```python
from build123d import *

# Parameters (mm, degrees)
BOSS_EXTRUDE3_DEPTH      = 4
BOSS_EXTRUDE3_DEPTH_BACK = 13
SKETCH1_R                = 2.5
SKETCH1_R_2              = 4.5
SKETCH1_R_3              = 2
SKETCH1_R_4              = 1
BOSS_EXTRUDE4_DEPTH      = 0.0001
BOSS_EXTRUDE4_DEPTH_BACK = 1
SKETCH1_3_R              = 1
SKETCH1_8_R              = 1
BOSS_EXTRUDE6_DEPTH      = 7
SKETCH1_9_R              = 2
BOSS_EXTRUDE7_DEPTH      = 11
SKETCH1_11_R             = 4.5
BOSS_EXTRUDE10_DEPTH     = 8
SKETCH1_12_R             = 4.5
SKETCH1_12_R_2           = 2.5
SKETCH1_12_R_3           = 1
BOSS_EXTRUDE11_DEPTH     = 6


with BuildPart() as part:
    # Sketch1 → Boss-Extrude3 (new, two sides: drawn at the far end of the back side and taken through both)
    # profile 1 of 14: a face of its own
    with BuildSketch(Plane(origin=(0, 0, 0), x_dir=(1, 0, 0), z_dir=(0, 1, 0)).offset(-BOSS_EXTRUDE3_DEPTH_BACK)):
        with BuildLine():
            ThreePointArc((-1.694444444, -2.401613398), (-3.327128661, -3.940638292), (-5.5, -4.5))
            Line((-5.5, -4.5), (10, -4.5))
            Line((10, -4.5), (10, 4.5))
            Line((10, 4.5), (-5.5, 4.5))
            ThreePointArc((-5.5, 4.5), (-3.327128661, 3.940638292), (-1.694444444, 2.401613398))
            ThreePointArc((-1.694444444, 2.401613398), (0.502313031, 1.998263135), (1.5, 0))
            ThreePointArc((1.5, 0), (0.502313031, -1.998263135), (-1.694444444, -2.401613398))
        make_face()
    # profile 2 of 14: a face of its own
    with BuildSketch(Plane(origin=(0, 0, 0), x_dir=(1, 0, 0), z_dir=(0, 1, 0)).offset(-BOSS_EXTRUDE3_DEPTH_BACK)):
        with BuildLine():
            Line((-10, 0), (-10, -4.5))
            Line((-10, -4.5), (-5.5, -4.5))
            ThreePointArc((-5.5, -4.5), (-8.681980515, -3.181980515), (-10, 0))
        make_face()
    # profile 3 of 14: a face of its own
    with BuildSketch(Plane(origin=(0, 0, 0), x_dir=(1, 0, 0), z_dir=(0, 1, 0)).offset(-BOSS_EXTRUDE3_DEPTH_BACK)):
        with BuildLine():
            Line((-10, 4.5), (-10, 0))
            ThreePointArc((-10, 0), (-8.681980515, 3.181980515), (-5.5, 4.5))
            Line((-5.5, 4.5), (-10, 4.5))
        make_face()
    # profile 4 of 14: a face of its own
    with BuildSketch(Plane(origin=(0, 0, 0), x_dir=(1, 0, 0), z_dir=(0, 1, 0)).offset(-BOSS_EXTRUDE3_DEPTH_BACK)):
        with Locations((-1, 0)):
            Circle(SKETCH1_R)
    # profile 5 of 14: a face of its own
    with BuildSketch(Plane(origin=(0, 0, 0), x_dir=(1, 0, 0), z_dir=(0, 1, 0)).offset(-BOSS_EXTRUDE3_DEPTH_BACK)):
        with Locations((-5.5, 0)):
            Circle(SKETCH1_R_2)
        with Locations((-5.5, 0)):
            Circle(SKETCH1_R_3, mode=Mode.SUBTRACT)
    # profile 6 of 14: a face of its own
    with BuildSketch(Plane(origin=(0, 0, 0), x_dir=(1, 0, 0), z_dir=(0, 1, 0)).offset(-BOSS_EXTRUDE3_DEPTH_BACK)):
        with Locations((-5.5, 0)):
            Circle(SKETCH1_R_3)
    # profile 7 of 14: a face of its own
    with BuildSketch(Plane(origin=(0, 0, 0), x_dir=(1, 0, 0), z_dir=(0, 1, 0)).offset(-BOSS_EXTRUDE3_DEPTH_BACK)):
        with Locations((-5.5, 0)):
            Circle(SKETCH1_R_2)
    # profile 8 of 14: a face of its own
    with BuildSketch(Plane(origin=(0, 0, 0), x_dir=(1, 0, 0), z_dir=(0, 1, 0)).offset(-BOSS_EXTRUDE3_DEPTH_BACK)):
        with Locations((-1, 0)):
            Circle(SKETCH1_R)
        with Locations((-1, 0)):
            Circle(SKETCH1_R_4, mode=Mode.SUBTRACT)
    # profile 9 of 14: a face of its own
    with BuildSketch(Plane(origin=(0, 0, 0), x_dir=(1, 0, 0), z_dir=(0, 1, 0)).offset(-BOSS_EXTRUDE3_DEPTH_BACK)):
        with Locations((-5.5, 0)):
            Circle(SKETCH1_R_2)
    # profile 10 of 14: a face of its own
    with BuildSketch(Plane(origin=(0, 0, 0), x_dir=(1, 0, 0), z_dir=(0, 1, 0)).offset(-BOSS_EXTRUDE3_DEPTH_BACK)):
        with Locations((-1, 0)):
            Circle(SKETCH1_R)
        with Locations((-1, 0)):
            Circle(SKETCH1_R_4, mode=Mode.SUBTRACT)
    # profile 11 of 14: a face of its own
    with BuildSketch(Plane(origin=(0, 0, 0), x_dir=(1, 0, 0), z_dir=(0, 1, 0)).offset(-BOSS_EXTRUDE3_DEPTH_BACK)):
        with Locations((-5.5, 0)):
            Circle(SKETCH1_R_2)
    # profile 12 of 14: a face of its own
    with BuildSketch(Plane(origin=(0, 0, 0), x_dir=(1, 0, 0), z_dir=(0, 1, 0)).offset(-BOSS_EXTRUDE3_DEPTH_BACK)):
        with Locations((-1, 0)):
            Circle(SKETCH1_R_4)
    # profile 13 of 14: a face of its own
    with BuildSketch(Plane(origin=(0, 0, 0), x_dir=(1, 0, 0), z_dir=(0, 1, 0)).offset(-BOSS_EXTRUDE3_DEPTH_BACK)):
        with Locations((-5.5, 0)):
            Circle(SKETCH1_R_2)
    # profile 14 of 14: a face of its own
    with BuildSketch(Plane(origin=(0, 0, 0), x_dir=(1, 0, 0), z_dir=(0, 1, 0)).offset(-BOSS_EXTRUDE3_DEPTH_BACK)):
        with Locations((-1, 0)):
            Circle(SKETCH1_R_4)
    extrude(amount=BOSS_EXTRUDE3_DEPTH + BOSS_EXTRUDE3_DEPTH_BACK)

    # Sketch1_3 → Boss-Extrude4 (add, two sides: drawn at the far end of the back side and taken through both)
    # profile 1 of 2: a face of its own
    with BuildSketch(Plane(origin=(0, 0, 0), x_dir=(1, 0, 0), z_dir=(0, 1, 0)).offset(-BOSS_EXTRUDE4_DEPTH_BACK)):
        with BuildLine():
            Line((-14, -4.5), (-10, -4.5))
            Line((-10, -4.5), (-10, 4.5))
            Line((-10, 4.5), (-14, 4.5))
            ThreePointArc((-14, 4.5), (-16.985823737, 0), (-14, -4.5))
        make_face()
        with Locations(Location((-13, 0, 0), (0, 0, 270))):
            Circle(SKETCH1_3_R, mode=Mode.SUBTRACT)
    # profile 2 of 2: a face of its own
    with BuildSketch(Plane(origin=(0, 0, 0), x_dir=(1, 0, 0), z_dir=(0, 1, 0)).offset(-BOSS_EXTRUDE4_DEPTH_BACK)):
        with BuildLine():
            Line((10, 4.5), (10, -4.5))
            Line((10, -4.5), (14, -4.5))
            ThreePointArc((14, -4.5), (17.054182563, 0), (14, 4.5))
            Line((14, 4.5), (10, 4.5))
        make_face()
        with Locations(Location((13, 0, 0), (0, 0, 270))):
            Circle(SKETCH1_3_R, mode=Mode.SUBTRACT)
    extrude(amount=BOSS_EXTRUDE4_DEPTH + BOSS_EXTRUDE4_DEPTH_BACK)

    # Sketch1_8 → Boss-Extrude6 (add)
    with BuildSketch(Plane(origin=(0, 0, 0), x_dir=(1, 0, 0), z_dir=(0, 1, 0))):
        with Locations(Location((-1, 0, 0), (0, 0, 270))):
            Circle(SKETCH1_8_R)
    extrude(amount=BOSS_EXTRUDE6_DEPTH)

    # Sketch1_9 → Boss-Extrude7 (add)
    with BuildSketch(Plane(origin=(0, 0, 0), x_dir=(1, 0, 0), z_dir=(0, 1, 0))):
        with Locations(Location((-5.5, 0, 0), (0, 0, 270))):
            Circle(SKETCH1_9_R)
    extrude(amount=BOSS_EXTRUDE7_DEPTH)

    # Sketch1_11 → Boss-Extrude10 (add)
    with BuildSketch(Plane(origin=(0, 0, 0), x_dir=(1, 0, 0), z_dir=(0, 1, 0))):
        with Locations(Location((-5.5, 0, 0), (0, 0, 270))):
            Circle(SKETCH1_11_R)
    extrude(amount=BOSS_EXTRUDE10_DEPTH)

    # Sketch1_12 → Boss-Extrude11 (add)
    # profile 1 of 8: a face of its own
    with BuildSketch(Plane(origin=(0, 0, 0), x_dir=(1, 0, 0), z_dir=(0, 1, 0))):
        with Locations(Location((-5.5, 0, 0), (0, 0, 270))):
            Circle(SKETCH1_12_R)
    # profile 2 of 8: a face of its own
    with BuildSketch(Plane(origin=(0, 0, 0), x_dir=(1, 0, 0), z_dir=(0, 1, 0))):
        with Locations((-1, 0)):
            Circle(SKETCH1_12_R_2)
        with Locations((-1, 0)):
            Circle(SKETCH1_12_R_3, mode=Mode.SUBTRACT)
    # profile 3 of 8: a face of its own
    with BuildSketch(Plane(origin=(0, 0, 0), x_dir=(1, 0, 0), z_dir=(0, 1, 0))):
        with Locations(Location((-5.5, 0, 0), (0, 0, 270))):
            Circle(SKETCH1_12_R)
    # profile 4 of 8: a face of its own
    with BuildSketch(Plane(origin=(0, 0, 0), x_dir=(1, 0, 0), z_dir=(0, 1, 0))):
        with Locations(Location((-5.5, 0, 0), (0, 0, 270))):
            Circle(SKETCH1_12_R)
    # profile 5 of 8: a face of its own
    with BuildSketch(Plane(origin=(0, 0, 0), x_dir=(1, 0, 0), z_dir=(0, 1, 0))):
        with Locations((-1, 0)):
            Circle(SKETCH1_12_R_2)
        with Locations((-1, 0)):
            Circle(SKETCH1_12_R_3, mode=Mode.SUBTRACT)
    # profile 6 of 8: a face of its own
    with BuildSketch(Plane(origin=(0, 0, 0), x_dir=(1, 0, 0), z_dir=(0, 1, 0))):
        with Locations((-1, 0)):
            Circle(SKETCH1_12_R_3)
    # profile 7 of 8: a face of its own
    with BuildSketch(Plane(origin=(0, 0, 0), x_dir=(1, 0, 0), z_dir=(0, 1, 0))):
        with Locations(Location((-5.5, 0, 0), (0, 0, 270))):
            Circle(SKETCH1_12_R)
    # profile 8 of 8: a face of its own
    with BuildSketch(Plane(origin=(0, 0, 0), x_dir=(1, 0, 0), z_dir=(0, 1, 0))):
        with Locations((-1, 0)):
            Circle(SKETCH1_12_R_3)
    extrude(amount=BOSS_EXTRUDE11_DEPTH)


solid = part.part
```
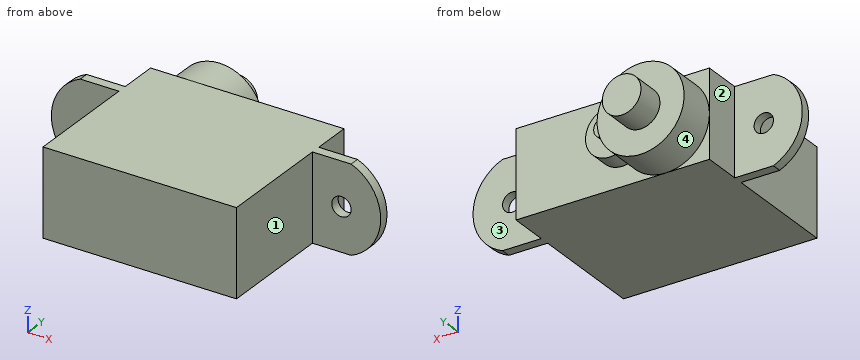
Check sheet for the modelled part. Datum: model origin and axes. Units: mm. Face numbers are marked on the shaded views. A direction names the side the tool comes from. Coordinates: 2 decimals unless noted, no trailing zeros. Write each loop counter-clockwise with the first axis right and the second up, starting at its lowest first coordinate (ties: lowest second). Pieces come first, ordered by that corner, then holes. Notation, with made-up numbers: (87, 83) -> (127, 83) arc R24 cw to (127, 102) -> close; hole circle Ø1 at (84.5, 7). An arc over 180 degrees is marked (long way). Use a Markdown table: item, result.
1. Sectioned sample at A-A (x = -13). Enter the section's corners in (y, z).
Reported:
| item | result |
|---|---|
| outline | (-1, -4.5) -> (0, -4.5) -> (0, -1) -> (-1, -1) -> close; (-1, 1) -> (0, 1) -> (0, 4.5) -> (-1, 4.5) -> close |
2. Go/stop test with flat-tipped pins: pin 1 Ø6 at (x, y) = (-10.5, 0.5) entering from +Z; pin 2 Ø3 at (x, z) = (-13, 0) entering from +Y; pin 3 Ø1.3 at (x, z) = (-8, 3.5) entering from +Y; pin 4 Ø4.5 at (y, z) = (-6.5, -1.5) entering from -X. Record where each tip stops, or that it passes through.
Reported:
| item | result |
|---|---|
| pin 1 | stops at z = 4.5 |
| pin 2 | stops at y = 0 |
| pin 3 | stops at y = 8 |
| pin 4 | stops at x = -10 |
3. Sectioned sample at C-C (y = -4.5). Enter the section's corners in (x, z).
Reported:
| item | result |
|---|---|
| outline | (-10, -4.5) -> (10, -4.5) -> (10, 4.5) -> (-10, 4.5) -> close |
4. Tool access check on the marked faces 1, 2, 3 and 4. Record the directions out of +Z, -Z, +X, -X, +Y, -Y that give a thin tool (end or side, any length) a straight path to the whole face; none if there is none.
Reported:
| item | result |
|---|---|
| face 1 | +Z, -Z, +X, -Y |
| face 2 | +Z, -Z, -X, +Y |
| face 3 | +Z, -Z, +X, +Y |
| face 4 | +Y |
5. Scan lines: line 1 along X through (y, z) = (-8.5, -1.75); line 2 along X through (y, z) = (8.75, 0); line 3 along Y through (x, z) = (13, -3). Record each from-to range of solid material in increasing order.
Reported:
| item | result |
|---|---|
| line 1 | x = -10 to 10 |
| line 2 | x = -7.5 to -3.5 |
| line 3 | y = -1 to 0 |
6. Sectioned sample at D-D (x = 12.5). Enter the section's corners in (y, z), plus the area to 3 significant figures.
Reported:
| item | result |
|---|---|
| outline | (-1, -4.5) -> (0, -4.5) -> (0, -0.87) -> (-1, -0.87) -> close; (-1, 0.87) -> (0, 0.87) -> (0, 4.5) -> (-1, 4.5) -> close |
| area | 7.27 mm2 |
